Read the model definition and answer for the solid it produces. Units are mm, in the model's axes. Face numbers are marked on the shaded views. Give positions to 0.01 mm unless a question says otherwise; leave off trailing zeros. Loops run counter-clockwise (first coordinate to the right, second up) from the corner with the lowest first, then second, coordinate; pieces in that order, holes last. Notation, with made-up numbers: (32, 13) - (63, 13) arc R38 ccw to (63, 52) - close; hole circle Ø7 at (79, -13.75). An arc over 180 degrees is marked (long way). Write item = value, one per line. Start each with the question number.
from build123d import *

# Parameters (mm, degrees)
SKETCH1_W                                  = 70
SKETCH1_H                                  = 115
BOSS_EXTRUDE1_DEPTH                        = 3
SKETCH4_R                                  = 2.25
CUT_EXTRUDE2_DEPTH                         = 3
MIRROR1_AT_THE_SECOND_PLANE_COPY_1_SKETC_R = 2.25
MIRROR1_AT_THE_SECOND_PLANE_COPY_1_DEPTH   = 3
FILLET4_R                                  = 1
CUT_EXTRUDE13_START                        = -3
CUT_EXTRUDE13_DEPTH                        = 4
SKETCH21_R                                 = 3
CUT_EXTRUDE14_DEPTH                        = 3


with BuildPart() as part:
    # Sketch1 → Boss-Extrude1 (new body)
    with BuildSketch(Plane(origin=(0, 0, 0), x_dir=(1, 0, 0), z_dir=(0, 1, 0))):
        Rectangle(SKETCH1_W, SKETCH1_H)
    extrude(amount=BOSS_EXTRUDE1_DEPTH)

    # Sketch4 → Cut-Extrude2 (cut)
    with BuildSketch(Plane(origin=(0, 0, 0), x_dir=(-1, 0, 0), z_dir=(0, -1, 0))):
        with Locations((30.5, -53)):
            Circle(SKETCH4_R)
    cut_extrude2 = extrude(amount=-CUT_EXTRUDE2_DEPTH, mode=Mode.SUBTRACT)

    # Mirror1: Cut-Extrude2 across plane
    add(cut_extrude2.mirror(Plane(origin=(0, 0, 0), x_dir=(0, 0, 1), z_dir=(1, 0, 0))), mode=Mode.SUBTRACT)

    # Mirror1 at the second plane: Cut-Extrude2 across plane
    add(cut_extrude2.mirror(Plane.XY), mode=Mode.SUBTRACT)

    # Mirror1 at the second plane copy 1 sketc → Mirror1 at the second plane copy 1 (cut)
    with BuildSketch(Plane.XZ):
        with Locations((30.5, -53)):
            Circle(MIRROR1_AT_THE_SECOND_PLANE_COPY_1_SKETC_R)
    extrude(amount=-MIRROR1_AT_THE_SECOND_PLANE_COPY_1_DEPTH, mode=Mode.SUBTRACT)

    # Fillet4
    fillet4_edges = [part.edges().sort_by_distance(p)[0] for p in [
        (0, 0, 57.5),
        (-35, 0, 0),
        (0, 0, -57.5),
        (35, 0, 0),
    ]]
    fillet(fillet4_edges, radius=FILLET4_R)

    # Sketch18 → Cut-Extrude13 (cut)
    with BuildSketch(Plane(origin=(0, 0, 0), x_dir=(-1, 0, 0), z_dir=(0, -1, 0)).offset(CUT_EXTRUDE13_START)):
        with BuildLine():
            Line((-9.797958971, -31.625), (9.797958971, -31.625))
            ThreePointArc((9.797958971, -31.625), (17.5, -17.125), (9.797958971, -2.625))
            Line((9.797958971, -2.625), (-9.797958971, -2.625))
            ThreePointArc((-9.797958971, -2.625), (-17.5, -17.125), (-9.797958971, -31.625))
        make_face()
    cut_extrude13 = extrude(amount=CUT_EXTRUDE13_DEPTH, mode=Mode.SUBTRACT)

    # Mirror3: Cut-Extrude13 across plane
    add(cut_extrude13.mirror(Plane.XY.offset(-2.525)), mode=Mode.SUBTRACT)

    # Sketch21 → Cut-Extrude14 (cut)
    with BuildSketch(Plane(origin=(0, 3, 0), x_dir=(1, 0, 0), z_dir=(0, 1, 0))):
        with Locations((0, 45.375)):
            Circle(SKETCH21_R)
        with Locations((0, -40.325)):
            Circle(SKETCH21_R)
    extrude(amount=-CUT_EXTRUDE14_DEPTH, mode=Mode.SUBTRACT)


solid = part.part
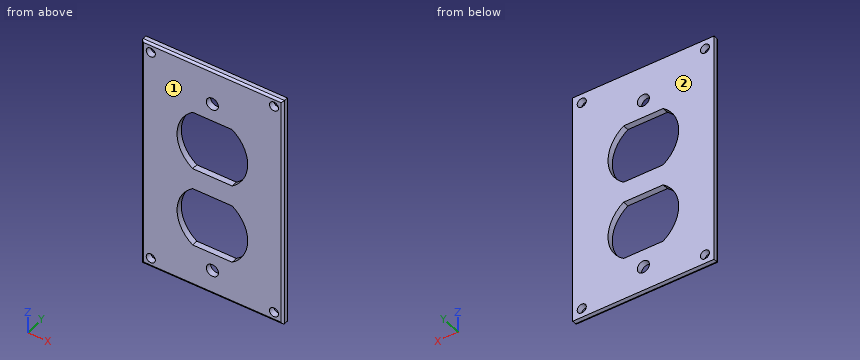
1. A cutting plane is placed at A-A on x = 5.5. Give the vertices of the cut face in (y, z) (3 decimals), and give its area (3 significant figures).
2. For a pull along Y with two mould halves and no side action, classify the marked faces 1 and 2 as released by +Y, released by -Y, zero draft, split by the parting line, or undercut.
3. A cutting plane is placed at D-D on y = 1.85. Give the number of separate pieces and of enclosed holes in the cut face, and give its area (3 significant figures).
4. Given P1, Ø3.5, axis at x = -30.5, z = 53, coming from the +Y side, flat-ended and moving along its own axis, determine where the tip first touches the part or whether it passes through.
5. A cutting plane is placed at B-B on z = 53. Give the vertices of the cut face in (x, y).
6. A cutting plane is placed at C-C on z = -43.5. Give the vertices of the cut face in (x, y).
7. Consider line 1 along Z through (x, y) = (9, 2.1) (3 decimals); line 2 along Z through (x, y) = (-30.5, 1.05); line 3 along X through (y, z) = (2.2, 53). Determine where each line is inside the solid, lowest interval first. Write a range as [from, to].
Reply:
q1.outline = (0, -56.5) arc R1 ccw to (1, -57.5) - (3, -57.5) - (3, -36.675) - (0, -36.675) - close; (0, -7.675) - (3, -7.675) - (3, 2.625) - (0, 2.625) - close; (0, 31.625) - (3, 31.625) - (3, 57.5) - (1, 57.5) arc R1 ccw to (0, 56.5) - close
q1.area = 171 mm^2
q2.face_1 = released by -Y
q2.face_2 = released by +Y
q3.separate_pieces = 1
q3.enclosed_holes = 8
q3.area = 6,170 mm^2
q4.P1 = through
q5.outline = (-35, 1) arc R1 ccw to (-34, 0) - (-32.75, 0) - (-32.75, 3) - (-35, 3) - close; (-28.25, 0) - (28.25, 0) - (28.25, 3) - (-28.25, 3) - close; (32.75, 0) - (34, 0) arc R1 ccw to (35, 1) - (35, 3) - (32.75, 3) - close
q6.outline = (-35, 1) arc R1 ccw to (-34, 0) - (-2.34, 0) - (-2.34, 3) - (-35, 3) - close; (2.34, 0) - (34, 0) arc R1 ccw to (35, 1) - (35, 3) - (2.34, 3) - close
q7.line_1 = [-57.5, -36.675], [-7.675, 2.625], [31.625, 57.5]
q7.line_2 = [-57.5, -55.25], [-50.75, 50.75], [55.25, 57.5]
q7.line_3 = [-35, -32.75], [-28.25, 28.25], [32.75, 35]
